Source: three-view drawing plus pictorial views. Frame: mm from the lowest corner of the part. A direction names the side the tool comes from. Give positions to 0.01 mm unless a question says otherwise; leave off trailing zeros. Loops run counter-clockwise (first coordinate to the right, second up) from the corner with the lowest first, then second, coordinate; pieces in that order, holes last.
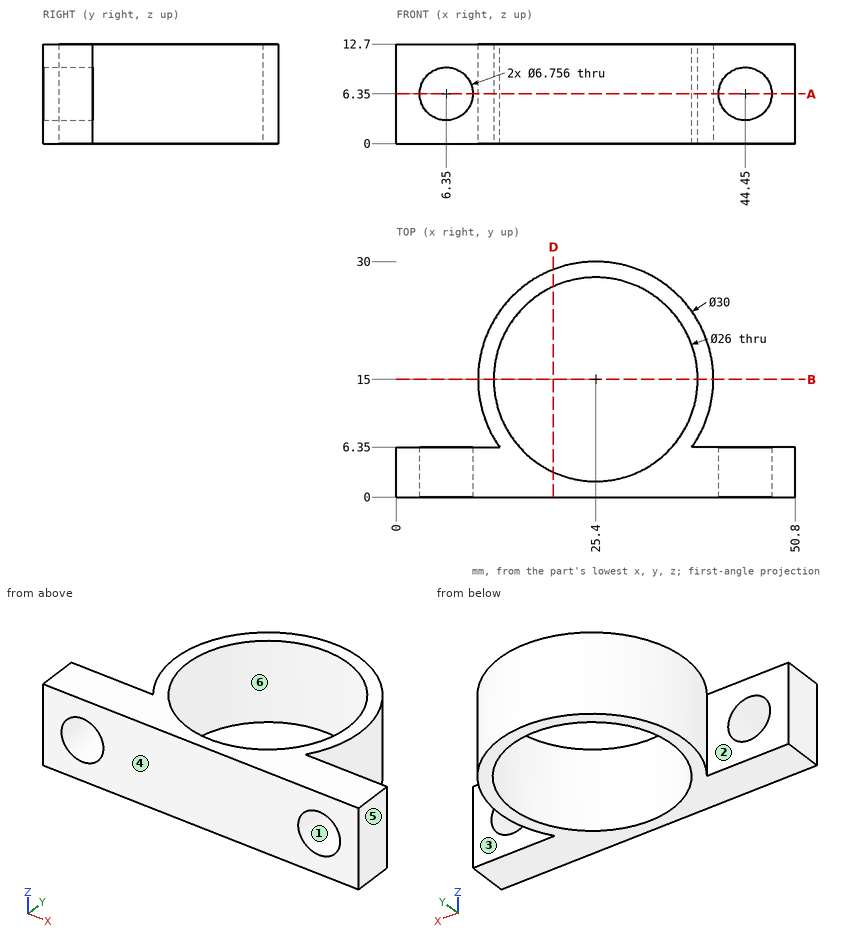
1) Cut plane D-D (x = 20). Return loops of the section in (y, z) (1 decimal).
Checks:
outline: (0, 0) - (3.2, 0) - (3.2, 12.7) - (0, 12.7) - close; (26.8, 0) - (29, 0) - (29, 12.7) - (26.8, 12.7) - close
2) Pull-direction query (Y, two-part tool) for the marked faces 4, 5 and 6; classes: released by +Y, released by -Y, zero draft, split by the parting line, or undercut.
Checks:
face 4: released by -Y
face 5: zero draft
face 6: undercut
3) Cut plane A-A (z = 6.35). State how many separate pieces and enclosed holes the cut face has.
Checks:
separate pieces: 3
enclosed holes: 1
4) Cut plane B-B (y = 15). Return loops of the section in (x, z).
Checks:
outline: (10.4, 0) - (12.4, 0) - (12.4, 12.7) - (10.4, 12.7) - close; (38.4, 0) - (40.4, 0) - (40.4, 12.7) - (38.4, 12.7) - close
5) Ray query, probe 1 along X at (y, z) = (14.5, 2.5); probe 2 along Z at (x, y) = (44.45, 2.5); probe 3 along Y at (x, z) = (25.4, 8.75). Return the intervals inside material, ascending.
Checks:
probe 1: x = 10.41 to 12.41, 38.39 to 40.39
probe 2: z = 0 to 2.97, 9.73 to 12.7
probe 3: y = 0 to 2, 28 to 30
6) Contact query for flat-ended pins moving along their axis: P1, Ø3, axis at y = 19, z = 5, coming from the +X side; P2, Ø4, axis at x = 44.5, z = 9, coming from the +Y side. Output: stop coordinate, or through.
Checks:
P1: stops at x = 40.19
P2: stops at y = 6.35
7) Reachability of the marked faces 1, 2 and 3 from +Z, -Z, +X, -X, +Y, -Y: full face, straight path, thin tool, end or side. Return the list, or none.
Checks:
face 1: +Y, -Y
face 2: +Z, -Z, -X
face 3: +Z, -Z, +X
